Read the model definition and answer for the solid it produces. Units are mm, in the model's axes. Round coordinates to 2 decimals unless told otherwise and drop trailing zeros. Order: outer loops, then holes, each group sorted by start corner. A loop starts at its lowest first (then second) coordinate and runs counter-clockwise, first axis right, second up. Notation, with made-up numbers: (68, 71) -> (104, 71) arc R32 ccw to (104, 97) -> close; hole circle Ø9 at (88, 89.25). An arc over 180 degrees is marked (long way). Answer as a JSON object with one key per item and string values. Group by question number.
Item 1: Section D-D, the plane y = 295 is taken. Write down the section's boundary in (x, z).
Item 2: Consider probe 1 along X at (y, z) = (304.5, 1.85); probe 2 along X at (y, z) = (240, 1.25); probe 3 along Y at (x, z) = (66, 1.5) (3 decimals). Determine where each line is inside the solid, lowest interval first. Write a range as from..to.
Item 3: Section C-C, the plane z = 2 is taken. Count the separate pieces of the cut face and the enclosed holes in it, plus the area to 3 significant figures.
Item 4: Section A-A, the plane y = 197 is taken. Write down the section's boundary in (x, z), plus the area to 3 significant figures.
Item 5: Section B-B, the plane x = -44.5 is taken. Write down the section's boundary in (y, z) (3 decimals).
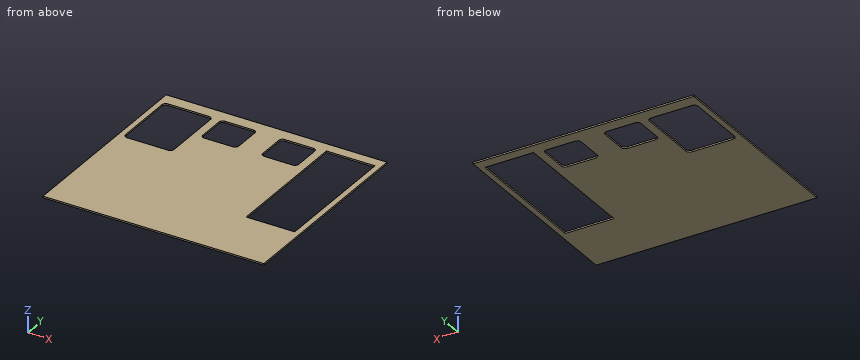
from build123d import *

# Parameters (mm, degrees)
SKETCH1_W                   = 82.55
SKETCH1_H                   = 223.52
BOSS_EXTRUDE1_DEPTH         = 2.667
CORNERRADIUSALLOWANCE_DEPTH = 408.419998422


with BuildPart() as part:
    # Sketch1 → Boss-Extrude1 (new body)
    with BuildSketch(Plane.XY):
        with BuildLine():
            Line((-193.04, 0), (-193.04, 349.25))
            ThreePointArc((-193.04, 349.25), (0, 358.775), (193.04, 349.25))
            Line((193.04, 349.25), (193.04, 0))
            Line((193.04, 0), (-193.04, 0))
        make_face()
        with BuildLine():
            Line((74.93, 264.795), (26.67, 264.795))
            ThreePointArc((26.67, 264.795), (22.179871939, 266.654871939), (20.32, 271.145))
            Line((20.32, 271.145), (20.32, 315.595))
            ThreePointArc((20.32, 315.595), (22.179871939, 320.085128061), (26.67, 321.945))
            Line((26.67, 321.945), (74.93, 321.945))
            ThreePointArc((74.93, 321.945), (79.420128061, 320.085128061), (81.28, 315.595))
            Line((81.28, 315.595), (81.28, 271.145))
            ThreePointArc((81.28, 271.145), (79.420128061, 266.654871939), (74.93, 264.795))
        make_face(mode=Mode.SUBTRACT)
        with BuildLine():
            Line((-171.45, 321.945), (-101.6, 321.945))
            ThreePointArc((-101.6, 321.945), (-97.109871939, 320.085128061), (-95.25, 315.595))
            Line((-95.25, 315.595), (-95.25, 213.995))
            ThreePointArc((-95.25, 213.995), (-97.109871939, 209.504871939), (-101.6, 207.645))
            Line((-101.6, 207.645), (-171.45, 207.645))
            ThreePointArc((-171.45, 207.645), (-175.940128061, 209.504871939), (-177.8, 213.995))
            Line((-177.8, 213.995), (-177.8, 315.595))
            ThreePointArc((-177.8, 315.595), (-175.940128061, 320.085128061), (-171.45, 321.945))
        make_face(mode=Mode.SUBTRACT)
        with BuildLine():
            Line((-74.93, 321.945), (-26.67, 321.945))
            ThreePointArc((-26.67, 321.945), (-22.179871939, 320.085128061), (-20.32, 315.595))
            Line((-20.32, 315.595), (-20.32, 271.145))
            ThreePointArc((-20.32, 271.145), (-22.179871939, 266.654871939), (-26.67, 264.795))
            Line((-26.67, 264.795), (-74.93, 264.795))
            ThreePointArc((-74.93, 264.795), (-79.420128061, 266.654871939), (-81.28, 271.145))
            Line((-81.28, 271.145), (-81.28, 315.595))
            ThreePointArc((-81.28, 315.595), (-79.420128061, 320.085128061), (-74.93, 321.945))
        make_face(mode=Mode.SUBTRACT)
        with Locations((136.525, 213.36)):
            Rectangle(SKETCH1_W, SKETCH1_H, mode=Mode.SUBTRACT)
    extrude(amount=BOSS_EXTRUDE1_DEPTH)

    # Sketch2 → CornerRadiusAllowance (cut, through all)
    with BuildSketch(Plane.XY.offset(2.667)):
        with BuildLine():
            Line((-187.198, 0), (-187.198, 342.9))
            Line((-187.198, 342.9), (0, 342.9))
            Line((0, 342.9), (0, 358.775))
            ThreePointArc((0, 358.775), (-96.63742446, 356.392302388), (-193.04, 349.25))
            Line((-193.04, 349.25), (-193.04, 0))
            Line((-193.04, 0), (-187.198, 0))
        make_face()
        with BuildLine():
            Line((0, 358.775), (0, 342.9))
            Line((0, 342.9), (187.198, 342.9))
            Line((187.198, 342.9), (187.198, 0))
            Line((187.198, 0), (193.04, 0))
            Line((193.04, 0), (193.04, 349.25))
            ThreePointArc((193.04, 349.25), (96.63742446, 356.392302388), (0, 358.775))
        make_face()
    extrude(amount=-CORNERRADIUSALLOWANCE_DEPTH, mode=Mode.SUBTRACT)


solid = part.part
Values found:
{
 "1": {"outline": "(-187.2, 0) -> (-177.8, 0) -> (-177.8, 2.67) -> (-187.2, 2.67) -> close; (-95.25, 0) -> (-81.28, 0) -> (-81.28, 2.67) -> (-95.25, 2.67) -> close; (-20.32, 0) -> (20.32, 0) -> (20.32, 2.67) -> (-20.32, 2.67) -> close; (81.28, 0) -> (95.25, 0) -> (95.25, 2.67) -> (81.28, 2.67) -> close; (177.8, 0) -> (187.2, 0) -> (187.2, 2.67) -> (177.8, 2.67) -> close"},
 "2": {"probe 1": "-187.2..-177.8, -95.25..-81.28, -20.32..20.32, 81.28..95.25, 177.8..187.2", "probe 2": "-187.2..-177.8, -95.25..95.25, 177.8..187.2", "probe 3": "0..264.795, 321.945..342.9"},
 "3": {"separate pieces": "1", "enclosed holes": "4", "area": "93,600 mm2"},
 "4": {"outline": "(-187.2, 0) -> (95.25, 0) -> (95.25, 2.67) -> (-187.2, 2.67) -> close; (177.8, 0) -> (187.2, 0) -> (187.2, 2.67) -> (177.8, 2.67) -> close", "area": "778 mm2"},
 "5": {"outline": "(0, 0) -> (264.795, 0) -> (264.795, 2.667) -> (0, 2.667) -> close; (321.945, 0) -> (342.9, 0) -> (342.9, 2.667) -> (321.945, 2.667) -> close"}
}
